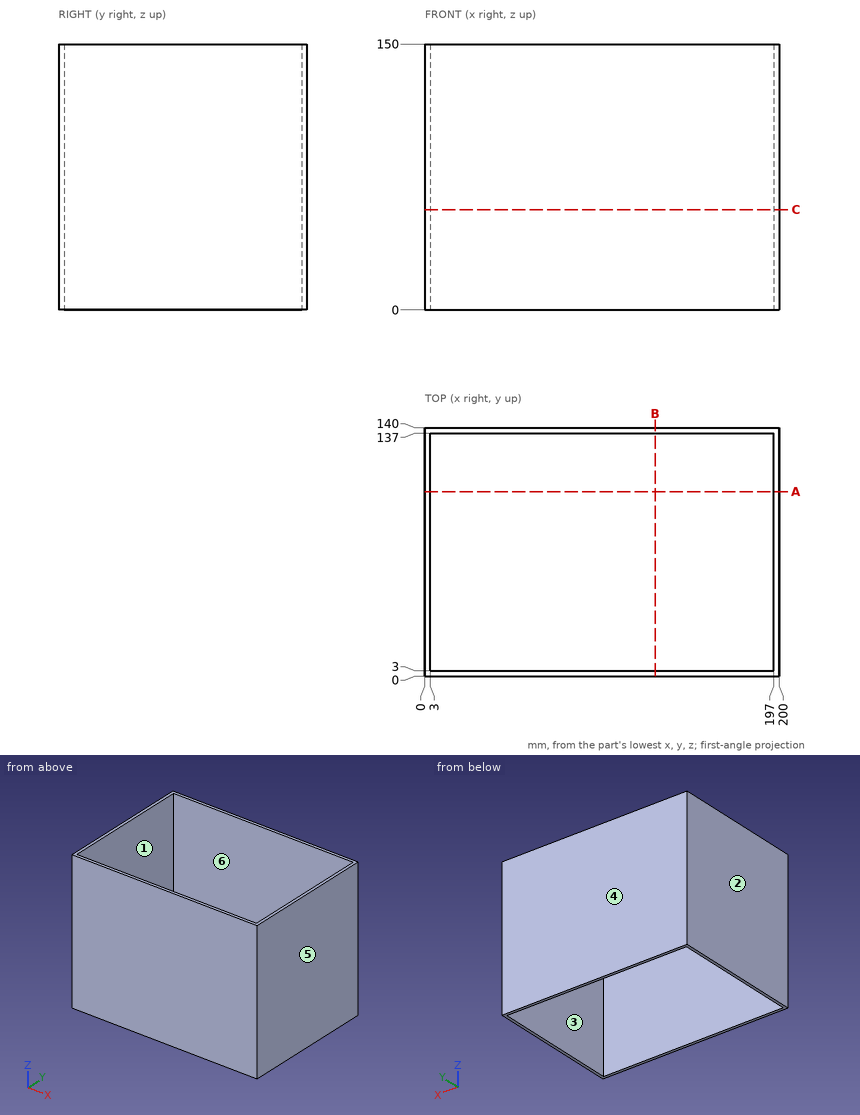
For this review, use the dimensioned drawing (mm, ordinates from the lowest corner) and the shaded views. A direction names the side the tool comes from. Coordinates: 2 decimals unless noted, no trailing zeros. Loops run counter-clockwise (first coordinate to the right, second up) from the corner with the lowest first, then second, coordinate; pieces in that order, holes last. Notation, with made-up numbers: (-32, 87) -> (27, 87) arc R27 ccw to (27, 123) -> close; hole circle Ø7 at (40, 85). An arc over 180 degrees is marked (long way). Return JSON: item names as keys, results as strings. Group by question number.
(1) Consider section C-C, the plane z = 56.5. Give the boundary of the cut face in (x, y), plus the area to 3 significant figures.
(2) Consider section A-A, the plane y = 104. Give the boundary of the cut face in (x, z).
(3) Tool access review of the marked faces 5 and 6: name each direction out of +Z, -Z, +X, -X, +Y, -Y from which nothing blocks a thin tool from reaching the whole face with its end or side.
(4) Consider section B-B, the plane x = 130. Give the boundary of the cut face in (y, z).
(5) Mouldability with a two-part tool opening along Y and no side actions: class the marked faces 1, 2, 3 and 4 as pulls with the +Y half, pulls with the -Y half, needs draft (parallel to the pull), parting line crosses it, or undercut.
(6) For pin 1 Ø6 at (y, z) = (62.5, 112) entering from -X, flat-tipped, find the tip position at first contact; note if it passes through.
(7) To check wall thickness, follow L1, parallel to Y at x = 151, z = 88; L2, parallel to X at y = 112.5, z = 142. State the ranges of each line that lie inside material, in increasing order.
Results below:
{
 "1": {"outline": "(0, 0) -> (200, 0) -> (200, 140) -> (0, 140) -> close; hole (3, 3) -> (197, 3) -> (197, 137) -> (3, 137) -> close", "area": "2,000 mm2"},
 "2": {"outline": "(0, 0) -> (3, 0) -> (3, 150) -> (0, 150) -> close; (197, 0) -> (200, 0) -> (200, 150) -> (197, 150) -> close"},
 "3": {"face 5": "+Z, -Z, +X, +Y, -Y", "face 6": "+Z, -Z"},
 "4": {"outline": "(0, 0) -> (3, 0) -> (3, 150) -> (0, 150) -> close; (137, 0) -> (140, 0) -> (140, 150) -> (137, 150) -> close"},
 "5": {"face 1": "undercut", "face 2": "needs draft", "face 3": "undercut", "face 4": "pulls with the +Y half"},
 "6": {"pin 1": "stops at x = 0"},
 "7": {"L1": "y = 0 to 3, 137 to 140", "L2": "x = 0 to 3, 197 to 200"}
}
